from build123d import *

# Parameters (mm, degrees)
BOSS_EXTRUDE1_DEPTH = 3


with BuildPart() as part:
    # Sketch1 → Boss-Extrude1 (new body)
    with BuildSketch(Plane.XY):
        with BuildLine():
            Line((-25, 0), (-15.5, 0))
            Line((-15.5, 0), (-14.5, 1))
            Line((-14.5, 1), (-14.5, 7.5))
            Line((-14.5, 7.5), (-10.5, 7.5))
            Line((-10.5, 7.5), (-10.5, 1))
            Line((-10.5, 1), (-9.5, 0))
            Line((-9.5, 0), (9.5, 0))
            Line((9.5, 0), (10.5, 1))
            Line((10.5, 1), (10.5, 7.5))
            Line((10.5, 7.5), (14.5, 7.5))
            Line((14.5, 7.5), (14.5, 1))
            Line((14.5, 1), (15.5, 0))
            Line((15.5, 0), (25, 0))
            ThreePointArc((25, 0), (18.922814713, 16.337903272), (3.645833333, 24.732729314))
            ThreePointArc((3.645833333, 24.732729314), (2.846483869, 24.50033273), (2.5, 23.743420141))
            Line((2.5, 23.743420141), (2.5, 17.5))
            Line((2.5, 17.5), (-1.5, 17.5))
            Line((-1.5, 17.5), (-1.5, 23.869436525))
            ThreePointArc((-1.5, 23.869436525), (-1.830734233, 24.612459629), (-2.604166667, 24.86399638))
            ThreePointArc((-2.604166667, 24.86399638), (-18.575577604, 16.731644171), (-25, 0))
        make_face()
    extrude(amount=BOSS_EXTRUDE1_DEPTH)


solid = part.part
Model file for the job. Use its own axes, mm. A direction names the side the tool comes from. Give positions to 0.01 mm unless a question says otherwise; leave off trailing zeros. Write each loop counter-clockwise with the first axis right and the second up, starting at its lowest first coordinate (ties: lowest second). Pieces come first, ordered by that corner, then holes. Notation, with made-up numbers: (-39, -12) -> (2, -12) arc R15 ccw to (2, -3) -> close; hole circle Ø10 at (-29, -14). An arc over 180 degrees is marked (long way). Write item = value, one per line.
(1) Slice it at A-A, the plane y = 4.75. Give the cut face in (x, z).
Determined:
outline = (-24.54, 0) -> (-14.5, 0) -> (-14.5, 3) -> (-24.54, 3) -> close; (-10.5, 0) -> (10.5, 0) -> (10.5, 3) -> (-10.5, 3) -> close; (14.5, 0) -> (24.54, 0) -> (24.54, 3) -> (14.5, 3) -> close
(2) Flat gauge pins, fed straight in: P1, Ø1, axis at y = 14.5, z = 2.5, coming from the +X side; P2, Ø1.5, axis at x = -0.5, z = 1.5, coming from the +Y side; P3, Ø2, axis at x = -11, y = 6.5, coming from the -Z side; P4, Ø1.5, axis at x = 19.5, z = 2.5, coming from the +Y side. Where does each tip first touch, or does it go through?
Determined:
P1 = 20.71
P2 = 17.5
P3 = 0
P4 = 16.54
(3) Slice it at B-B, the plane z = 0.5. Give the cut face in (x, y).
Determined:
outline = (-25, 0) -> (-15.5, 0) -> (-14.5, 1) -> (-14.5, 7.5) -> (-10.5, 7.5) -> (-10.5, 1) -> (-9.5, 0) -> (9.5, 0) -> (10.5, 1) -> (10.5, 7.5) -> (14.5, 7.5) -> (14.5, 1) -> (15.5, 0) -> (25, 0) arc R25 ccw to (3.65, 24.73) arc R1 ccw to (2.5, 23.74) -> (2.5, 17.5) -> (-1.5, 17.5) -> (-1.5, 23.87) arc R1 ccw to (-2.6, 24.86) arc R25 ccw to start
(4) Tool access for faces 1 (the face through (19.085, 16.148, 1.479)), 2 (the face through (2.5, 21, 1)), 3 (the face through (-13, 7.5, 1)): list every direction of +Z, -Z, +X, -X, +Y, -Y with a clear straight run to the whole face (end or side of a thin tool).
Determined:
face_1 = +Z, -Z, +X, +Y
face_2 = +Z, -Z, +Y
face_3 = +Z, -Z, -Y
(5) Mould opens along X. For faces 4 (the face through (0, 10, 3)), 5 (the face through (12, 7.5, 1)), 6 (the face through (2.86, 24.51, 1.48)), 7 (the face through (-18.403, 16.921, 1.479)) say: released by +X, released by -X, zero draft, split by the parting line, or undercut.
Determined:
face_4 = zero draft
face_5 = undercut
face_6 = undercut
face_7 = released by -X
(6) Slice it at C-C, the plane x = -9. Give the cut face in (y, z).
Determined:
outline = (0, 0) -> (23.32, 0) -> (23.32, 3) -> (0, 3) -> close
(7) Slice it at D-D, the plane y = 15. Give the cut face in (x, z), then the cut area to 3 significant figures.
Determined:
outline = (-20, 0) -> (20, 0) -> (20, 3) -> (-20, 3) -> close
area = 120 mm2
(8) Probe line 1 along X through (y, z) = (2, 2.4); line 2 along X through (y, z) = (18.5, 1.95); line 3 along X through (y, z) = (3.5, 2.85). List the from-to ranges inside material, lowest first.
Determined:
line_1 = -24.92 to -14.5, -10.5 to 10.5, 14.5 to 24.92
line_2 = -16.82 to -1.5, 2.5 to 16.82
line_3 = -24.75 to -14.5, -10.5 to 10.5, 14.5 to 24.75
